```python
from build123d import *

# Parameters (mm, degrees)
SKETCH1_R                   = 6.35
BOSS_EXTRUDE1_DEPTH         = 78.2574
F_1_4_20_TAPPED_HOLE1_D     = 5.1054
F_1_4_20_TAPPED_HOLE1_DEPTH = 40
F_1_4_20_TAPPED_HOLE1_TIP   = 1.533816902
F_1_4_20_TAPPED_HOLE2_D     = 5.1054
F_1_4_20_TAPPED_HOLE2_DEPTH = 40
F_1_4_20_TAPPED_HOLE2_TIP   = 1.533816902
CHAMFER1_SIZE               = 0.254


with BuildPart() as part:
    # Sketch1 → Boss-Extrude1 (new body, symmetric)
    with BuildSketch(Plane.XY):
        Circle(SKETCH1_R)
    extrude(amount=BOSS_EXTRUDE1_DEPTH, both=True)

    # 1/4-20 Tapped Hole1
    with Locations(Plane.XY.offset(78.2574)):
        with Locations((0, 0)):
            Hole(F_1_4_20_TAPPED_HOLE1_D / 2, depth=F_1_4_20_TAPPED_HOLE1_DEPTH)
            with Locations((0, 0, -(F_1_4_20_TAPPED_HOLE1_DEPTH + F_1_4_20_TAPPED_HOLE1_TIP / 2))):  # 118° drill point
                Cone(0, F_1_4_20_TAPPED_HOLE1_D / 2, F_1_4_20_TAPPED_HOLE1_TIP, mode=Mode.SUBTRACT)

    # 1/4-20 Tapped Hole2
    with Locations(Plane(origin=(0, 0, -78.2574), x_dir=(-1, 0, 0), z_dir=(0, 0, -1))):
        with Locations((0, 0)):
            Hole(F_1_4_20_TAPPED_HOLE2_D / 2, depth=F_1_4_20_TAPPED_HOLE2_DEPTH)
            with Locations((0, 0, -(F_1_4_20_TAPPED_HOLE2_DEPTH + F_1_4_20_TAPPED_HOLE2_TIP / 2))):  # 118° drill point
                Cone(0, F_1_4_20_TAPPED_HOLE2_D / 2, F_1_4_20_TAPPED_HOLE2_TIP, mode=Mode.SUBTRACT)

    # Chamfer1
    chamfer1_edges = [part.edges().sort_by_distance(p)[0] for p in [
        (-6.35, 0, -78.2574),
        (-6.35, 0, 78.2574),
    ]]
    chamfer(chamfer1_edges, length=CHAMFER1_SIZE)


solid = part.part
```
For this review, take the finished solid that the model builds, in its own axes (mm). A direction names the side the tool comes from. Coordinates: 2 decimals unless noted, no trailing zeros. Loops run counter-clockwise (first coordinate to the right, second up) from the corner with the lowest first, then second, coordinate; pieces in that order, holes last. Notation, with made-up numbers: (18.5, -19.75) - (74.5, -19.75) arc R16 cw to (74.5, 2.25) - close; hole circle Ø9 at (-15, -9.5). An arc over 180 degrees is marked (long way). Use one line per item in the form item = value. Start each with the question number.
1) Take a section at B-B (z = 19.5). State the section outline as (x, y) points, plus the area to 3 significant figures.
2) Take a section at A-A (z = -68.5). State the section outline as (x, y) points.
3) To check wall thickness, follow probe 1 along Y at (x, z) = (0, -65.5); probe 2 along X at (y, z) = (0.25, 47); probe 3 along Y at (x, z) = (1.75, 66). State the ranges of each line that lie inside material, in increasing order. Write a range as from..to.
4) For faces 5 (the face through (-2.435, 0.767, 57.977)), 6 (the face through (3, 0, -78.257)), list the 3-axis set-ups (+Z, -Z, +X, -X, +Y, -Y) from which the entire face can be reached by the end or side of a thin tool; tool diameter is ignored.
5) Draft analysis for pull direction X (two halves, no side actions). For faces 1 (the face through (3, 0, 78.257)), 2 (the face through (2.435, 0.767, -57.977)), 3 (the face through (-0.42, 0.13, -36.99)), 4 (the face through (-1.38, -6.2, 1.09)), state which applies: released by +X, released by -X, zero draft, split by the parting line, or undercut.
6) For pin 1 (1.5 mm diameter, centred on y = 3.5, z = -15.5, fed in from +X); pin 2 (1.5 mm diameter, centred on x = 3.5, z = 1, fed in from +Y); pin 3 (5 mm diameter, centred on y = -5, z = -15, fed in from +X), all flat-tipped, find the tip position at first contact; note any pin that passes through.
From the geometry:
q1.outline = circle Ø12.7 at (0, 0)
q1.area = 127 mm2
q2.outline = circle Ø12.7 at (0, 0); hole circle Ø5.11 at (0, 0)
q3.probe_1 = -6.35..-2.55, 2.55..6.35
q3.probe_2 = -6.35..-2.54, 2.54..6.35
q3.probe_3 = -6.1..-1.86, 1.86..6.1
q4.face_5 = +Z
q4.face_6 = -Z, +X, -X, +Y, -Y
q5.face_1 = zero draft
q5.face_2 = undercut
q5.face_3 = undercut
q5.face_4 = split by the parting line
q6.pin_1 = 5.72
q6.pin_2 = 5.72
q6.pin_3 = 5.84
